from build123d import *

# Parameters (mm, degrees)
SKETCH1_W           = 10
SKETCH1_H           = 15
BOSS_EXTRUDE1_DEPTH = 10
FILLET1_R           = 2
FILLET2_R           = 5


with BuildPart() as part:
    # Sketch1 → Boss-Extrude1 (new body)
    with BuildSketch(Plane(origin=(0, 0, 0), x_dir=(1, 0, 0), z_dir=(0, 1, 0))):
        with Locations((4.913793103, 7.456896552)):
            Rectangle(SKETCH1_W, SKETCH1_H)
        Polygon((19.913793103, 14.956896552), (4.913793103, 24.956896552), (4.913793103, 14.956896552), (9.913793103, 14.956896552), align=None)
        Polygon((4.913793103, 24.956896552), (-10.086206897, 14.956896552), (-0.086206897, 14.956896552), (4.913793103, 14.956896552), align=None)
    extrude(amount=BOSS_EXTRUDE1_DEPTH)

    # Fillet1
    fillet1_edges = [part.edges().sort_by_distance(p)[0] for p in [
        (-10.086206897, 5, -14.956896552),
        (19.913793103, 5, -14.956896552),
    ]]
    fillet(fillet1_edges, radius=FILLET1_R)

    # Fillet2
    fillet2_edges = [part.edges().sort_by_distance(p)[0] for p in [
        (4.913793103, 5, -24.956896552),
    ]]
    fillet(fillet2_edges, radius=FILLET2_R)


solid = part.part
Verification items for the finished model (mm, model axes). A direction names the side the tool comes from. Give positions to 0.01 mm unless a question says otherwise; leave off trailing zeros. Write each loop counter-clockwise with the first axis right and the second up, starting at its lowest first coordinate (ties: lowest second). Pieces come first, ordered by that corner, then holes.
(1) Gauge pin test, flat ends, axial feed: pin 1 (5 mm diameter, centred on y = 3, z = -6, fed in from +X); pin 2 (1.5 mm diameter, centred on y = 7.5, z = -11.5, fed in from -X); pin 3 (1.7 mm diameter, centred on x = -2, y = 4, fed in from +Z). Record the tip position at first contact, or that the pin passes through.
(2) Mould release check, pull along X, two halves, no side actions. Record for faces 1 (the face through (9.914, 5, -7)), 2 (the face through (-1.178, 4.93, -20.896)), 3 (the face through (4.955, 5.07, -23.947)), 4 (the face through (-2, 5, -14.957)): +X half, -X half, draft (parallel to the pull), parting line (faces both ways), or undercut.
(3) Cross-section at B-B (z = -20.25). Enter the section's corners in (x, y).
(4) Cross-section at C-C (x = -2.75). Enter the section's corners in (y, z).
(5) Material ranges on line 1 (X direction, y = 7.5, z = -8.5); line 2 (X direction, y = 1, z = -16.5); line 3 (Z direction, x = 9.75, y = 8.5), recorded low to high.
(6) Access from +Z, -Z, +X, -X, +Y, -Y to the whole of each face (thin tool, end or side, straight path). Record for faces 5 (the face through (-0.086, 5, -7)), 6 (the face through (5, 0, -12)), 7 (the face through (12, 5, -14.957)).
(7) Cross-section at A-A (y = 8). Enter the section's corners in (x, z).
Worked out:
1. pin 1: stops at x = 9.91
1. pin 2: stops at x = -0.09
1. pin 3: stops at z = -14.96
2. face 1: +X half
2. face 2: -X half
2. face 3: parting line
2. face 4: draft
3. outline: (-2.15, 0) - (11.97, 0) - (11.97, 10) - (-2.15, 10) - close
4. outline: (0, -19.85) - (10, -19.85) - (10, -14.96) - (0, -14.96) - close
5. line 1: x = -0.09 to 9.91
5. line 2: x = -5.43 to 15.26
5. line 3: z = -21.73 to 0.04
6. face 5: +Z, -X, +Y, -Y
6. face 6: +Z, -Z, +X, -X, -Y
6. face 7: +Z, +X, +Y, -Y
7. outline: (-4.59, -18.62) - (2.14, -23.11) arc R5 ccw to (7.69, -23.11) - (14.42, -18.62) arc R2 ccw to (13.31, -14.96) - (9.91, -14.96) - (9.91, 0.04) - (-0.09, 0.04) - (-0.09, -14.96) - (-3.48, -14.96) arc R2 ccw to start
